```python
from build123d import *

# Parameters (mm, degrees)
BOSS_EXTRUDE1_DEPTH = 30
FILLET1_R           = 3
FILLET2_R           = 0.5
FILLET3_R           = 1
CUT_EXTRUDE1_DEPTH  = 10


with BuildPart() as part:
    # Sketch1 → Boss-Extrude1 (new body)
    with BuildSketch(Plane.XY):
        Polygon((0, 0), (0, 50), (12.5, 50), (12.5, 25), (10.5, 25), (10.5, 48), (6.7, 48), (4, 43.5), (4, 0), align=None)
    extrude(amount=BOSS_EXTRUDE1_DEPTH)

    # Fillet1
    fillet1_edges = [part.edges().sort_by_distance(p)[0] for p in [
        (0, 50, 15),
        (12.5, 50, 15),
    ]]
    fillet(fillet1_edges, radius=FILLET1_R)

    # Fillet2
    fillet2_edges = [part.edges().sort_by_distance(p)[0] for p in [
        (10.5, 48, 15),
    ]]
    fillet(fillet2_edges, radius=FILLET2_R)

    # Fillet3
    fillet3_edges = [part.edges().sort_by_distance(p)[0] for p in [
        (12.5, 25, 15),
    ]]
    fillet(fillet3_edges, radius=FILLET3_R)

    # Sketch2 → Cut-Extrude1 (cut)
    with BuildSketch(Plane.ZY):
        Polygon((10, 42), (20, 42), (18, 36), (30, 36), (30, 0), (0, 0), (0, 36), (12, 36), align=None)
    extrude(amount=-CUT_EXTRUDE1_DEPTH, mode=Mode.SUBTRACT)


solid = part.part
```
Check sheet for the modelled part. Datum: model origin and axes. Units: mm. A direction names the side the tool comes from. Give positions to 0.01 mm unless a question says otherwise; leave off trailing zeros. Write each loop counter-clockwise with the first axis right and the second up, starting at its lowest first coordinate (ties: lowest second). Pieces come first, ordered by that corner, then holes.
Item 1: Draft check along Y on faces 6 (the face through (2, 39, 19)), 7 (the face through (0.86, 49.1, 15.21)), 8 (the face through (4, 42.3, 14.8)). Enter one of: released by +Y, released by -Y, zero draft, split by the parting line, or undercut.
Item 2: Cross-section at B-B (z = 19.5). Enter the section's corners in (x, y), and give its area (3 significant figures).
Item 3: Cross-section at C-C (z = 14.25). Enter the section's corners in (x, y).
Item 4: Scan lines: L1, parallel to X at y = 43.25, z = 4.25; L2, parallel to X at y = 44.5, z = 13.25; L3, parallel to Y at x = 3, z = 22.25. Record each from-to range of solid material in increasing order.
Item 5: Access from +Z, -Z, +X, -X, +Y, -Y to the whole of each face (thin tool, end or side, straight path). Record for faces 1 (the face through (2, 39, 11)), 2 (the face through (12.5, 37, 15)), 3 (the face through (11, 40, 30)), 4 (the face through (10.5, 36, 15)), 5 (the face through (2, 36, 24)).
Item 6: Gauge pin test, flat ends, axial feed: pin 1 (4.5 mm diameter, centred on x = 2, z = 16, fed in from -Y); pin 2 (3.5 mm diameter, centred on x = 8, z = 14.5, fed in from -Y). Record the tip position at first contact, or that the pin passes through.
Item 7: Cross-section at D-D (x = 2). Enter the section's corners in (y, z).
Item 8: Cross-section at A-A (y = 39). Enter the section's corners in (x, z), and give its area (3 significant figures).
Report:
1. face 6: undercut
1. face 7: released by +Y
1. face 8: zero draft
2. outline: (0, 36) - (4, 36) - (4, 40.5) - (0, 40.5) - close; (0, 42) - (4, 42) - (4, 43.5) - (6.7, 48) - (10, 48) arc R0.5 cw to (10.5, 47.5) - (10.5, 25) - (11.5, 25) arc R1 ccw to (12.5, 26) - (12.5, 47) arc R3 ccw to (9.5, 50) - (3, 50) arc R3 ccw to (0, 47) - close
2. area: 115 mm2
3. outline: (0, 42) - (4, 42) - (4, 43.5) - (6.7, 48) - (10, 48) arc R0.5 cw to (10.5, 47.5) - (10.5, 25) - (11.5, 25) arc R1 ccw to (12.5, 26) - (12.5, 47) arc R3 ccw to (9.5, 50) - (3, 50) arc R3 ccw to (0, 47) - close
4. L1: x = 0 to 4, 10.5 to 12.5
4. L2: x = 0 to 4.6, 10.5 to 12.5
4. L3: y = 36 to 50
5. face 1: -X
5. face 2: +Z, -Z, +X, +Y, -Y
5. face 3: +Z, +X, -X, +Y, -Y
5. face 4: +Z, -Z, -Y
5. face 5: +Z, -Z, -X, -Y
6. pin 1: stops at y = 36
6. pin 2: stops at y = 47.25
7. outline: (36, 0) - (49.83, 0) - (49.83, 30) - (36, 30) - (36, 18) - (42, 20) - (42, 10) - (36, 12) - close
8. outline: (0, 0) - (4, 0) - (4, 11) - (0, 11) - close; (0, 19) - (4, 19) - (4, 30) - (0, 30) - close; (10.5, 0) - (12.5, 0) - (12.5, 30) - (10.5, 30) - close
8. area: 148 mm2
